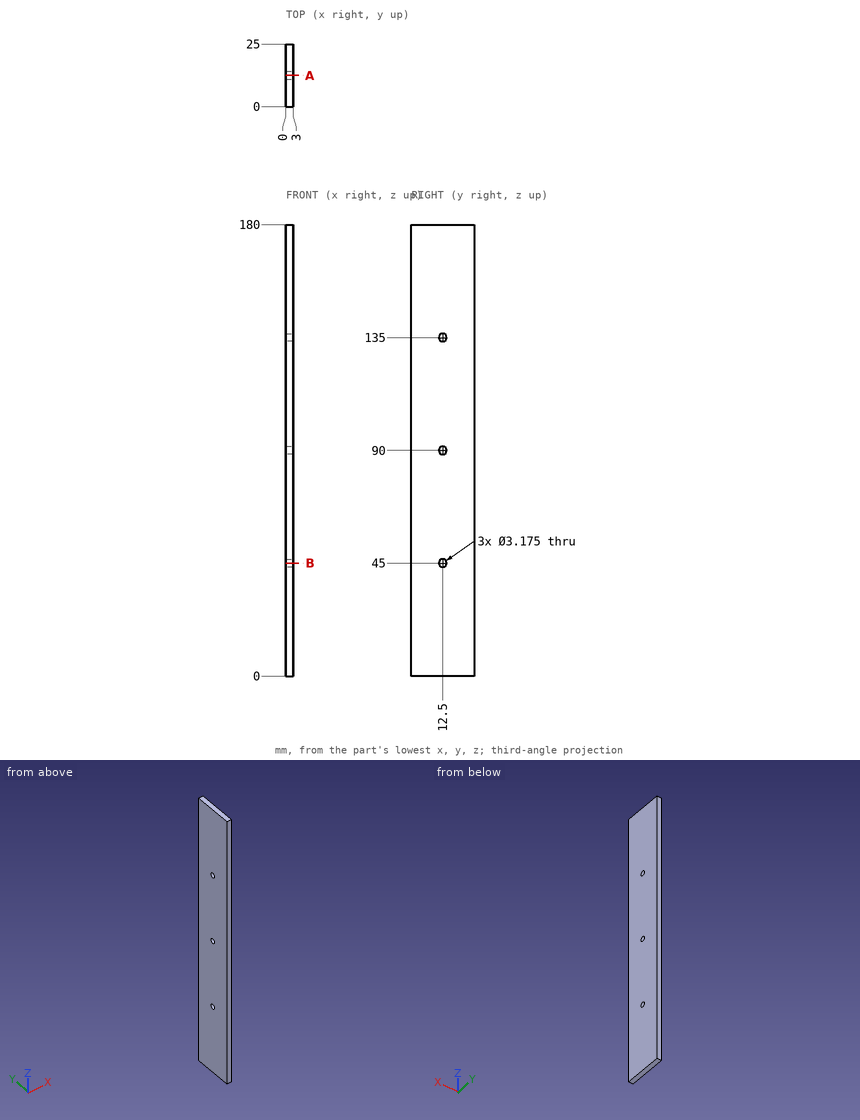
Check sheet for the drawn part. Datum: minimum x, y, z corner. Units: mm. Coordinates: 2 decimals unless noted, no trailing zeros. Write each loop counter-clockwise with the first axis right and the second up, starting at its lowest first coordinate (ties: lowest second). Pieces come first, ordered by that corner, then holes. Notation, with made-up numbers: (69.25, 1.25) - (94.25, 1.25) arc R27 ccw to (94.25, 31.25) - close; hole circle Ø9 at (87, 32). An arc over 180 degrees is marked (long way). Answer as a JSON object with one key per item and string values.
(1) Gauge pin test, flat end, axial feed: pin 1 Ø3.5 at (y, z) = (12.5, 135) entering from -X. Record the tip position at first contact, or that the pin passes through.
Report:
{"pin 1": "x = 0"}
(2) Cross-section at A-A on y = 12.5. Record the cut outline in (x, z).
Report:
{"outline": "(0, 0) - (3, 0) - (3, 43.41) - (0, 43.41) - close; (0, 46.59) - (3, 46.59) - (3, 88.41) - (0, 88.41) - close; (0, 91.59) - (3, 91.59) - (3, 133.41) - (0, 133.41) - close; (0, 136.59) - (3, 136.59) - (3, 180) - (0, 180) - close"}
(3) Cross-section at B-B on z = 45. Record the cut outline in (x, y), plus the area to 3 significant figures.
Report:
{"outline": "(0, 0) - (3, 0) - (3, 10.91) - (0, 10.91) - close; (0, 14.09) - (3, 14.09) - (3, 25) - (0, 25) - close", "area": "65.5 mm^2"}
(4) Thickness scan on line 1 along Y through (x, z) = (1.55, 45); line 2 along Z through (x, y) = (0.6, 12). Record the ranges inside material, lowest first.
Report:
{"line 1": "0 to 10.91, 14.09 to 25", "line 2": "0 to 43.49, 46.51 to 88.49, 91.51 to 133.49, 136.51 to 180"}
